from build123d import *

# Parameters (mm, degrees)
MODEL_R                 = 1.7
MODEL_R_2               = 1.600279216
MODEL_W                 = 3.1
MODEL_H                 = 6
SALIENTE_EXTRUIR1_DEPTH = 3


with BuildPart() as part:
    # Model → Saliente-Extruir1 (new body)
    with BuildSketch(Plane.XY):
        with BuildLine():
            Line((139.768153306, -45.054934941), (61.763543448, -45.054934941))
            ThreePointArc((61.763543448, -45.054934941), (60.702883276, -45.494274769), (60.263543448, -46.554934941))
            Line((60.263543448, -46.554934941), (60.263543448, -115.557339175))
            ThreePointArc((60.263543448, -115.557339175), (60.702883276, -116.617999347), (61.763543448, -117.057339175))
            Line((61.763543448, -117.057339175), (139.768153306, -117.057339175))
            ThreePointArc((139.768153306, -117.057339175), (140.828813478, -116.617999347), (141.268153306, -115.557339175))
            Line((141.268153306, -115.557339175), (141.268153306, -46.554934941))
            ThreePointArc((141.268153306, -46.554934941), (140.828813478, -45.494274769), (139.768153306, -45.054934941))
        make_face()
        with Locations((136.768487808, -103.558008179)):
            Circle(MODEL_R, mode=Mode.SUBTRACT)
        with Locations((136.768487808, -58.554600438)):
            Circle(MODEL_R, mode=Mode.SUBTRACT)
        with Locations((136.768487808, -112.557673677)):
            Circle(MODEL_R_2, mode=Mode.SUBTRACT)
        with Locations((136.768487808, -49.554934941)):
            Circle(MODEL_R_2, mode=Mode.SUBTRACT)
        with Locations((64.763543448, -103.558008179)):
            Circle(MODEL_R, mode=Mode.SUBTRACT)
        with Locations((64.763543448, -58.554600438)):
            Circle(MODEL_R, mode=Mode.SUBTRACT)
        with Locations((64.763543448, -49.554934941)):
            Circle(MODEL_R_2, mode=Mode.SUBTRACT)
        with Locations((64.763543448, -112.557673677)):
            Circle(MODEL_R_2, mode=Mode.SUBTRACT)
        with Locations((80.876831082, -110.067386969)):
            Rectangle(MODEL_W, MODEL_H, mode=Mode.SUBTRACT)
        with Locations((88.022204789, -110.067386969)):
            Rectangle(MODEL_W, MODEL_H, mode=Mode.SUBTRACT)
        Polygon((63.351345037, -62.275422733), (63.351345037, -72.689428622), (63.251345037, -72.789428622), (62.088360478, -72.789428622), (61.988360478, -72.889428622), (61.988360478, -76.624152209), (62.088360478, -76.724152209), (62.251345037, -76.724152209), (62.351345037, -76.824152209), (62.351345037, -99.677826967), (63.351345037, -99.677826967), (64.151345037, -100.477826967), (66.651345037, -100.477826967), (67.151345037, -100.977826967), (67.151345037, -114.477826967), (67.651345037, -114.977826967), (77.980472194, -114.977826967), (77.980472194, -106.277895967), (78.980472194, -105.277865819), (90.361604846, -105.277522697), (91.361604845, -106.277492548), (91.361604845, -114.977826967), (133.468205597, -114.977826967), (133.968205597, -114.477826967), (133.968205597, -100.862451961), (134.355954895, -100.477826967), (137.555954895, -100.477826967), (139.366374234, -98.667407629), (139.366374234, -61.475422733), (138.866374234, -60.975422733), (133.634687553, -60.975422733), (132.355954895, -60.088974267), (132.355954895, -48.775422733), (130.555954895, -46.975422733), (71.151345037, -46.975422733), (69.351345037, -48.775422733), (69.351345037, -58.538415371), (67.351345037, -61.475422733), (64.151345037, -61.475422733), align=None, mode=Mode.SUBTRACT)
    extrude(amount=SALIENTE_EXTRUIR1_DEPTH)


solid = part.part
Work out the finished part from the listing and answer in its coordinate system (mm). A direction names the side the tool comes from. Round coordinates to 2 decimals unless told otherwise and drop trailing zeros. Write each loop counter-clockwise with the first axis right and the second up, starting at its lowest first coordinate (ties: lowest second). Pieces come first, ordered by that corner, then holes. Notation, with made-up numbers: M 12.5,58 L 36.5,58 A21 ccw 36.5,70 Z; hole C 23,-4.5 d5. An arc over 180 degrees is marked long. Use a Markdown table: item, result.
1) The part is cut by section D-D on z = 2.1. State how many separate pieces and enclosed holes the cut face has, plus the area to 3 significant figures.
Taken from the geometry:
| item | result |
|---|---|
| separate pieces | 1 |
| enclosed holes | 11 |
| area | 977 mm2 |
2) Consider line 1 (Y direction, x = 88.5, z = 1.1); line 2 (X direction, y = -93, z = 2.6); line 3 (Y direction, x = 113, z = 0.45). Determine where each line is inside the solid, lowest interval first. Write a range as [from, to].
Taken from the geometry:
| item | result |
|---|---|
| line 1 | y = [-117.06, -113.07], [-107.07, -105.28], [-46.98, -45.05] |
| line 2 | x = [60.26, 62.35], [139.37, 141.27] |
| line 3 | y = [-117.06, -114.98], [-46.98, -45.05] |
3) Which of the six approach directions +Z, -Z, +X, -X, +Y, -Y give full straight-line access (tool end or side, diameter ignored) to faces 4 (the face through (101, -45.055, 1)), 5 (the face through (91.362, -111, 1))?
Taken from the geometry:
| item | result |
|---|---|
| face 4 | +Z, -Z, +X, -X, +Y |
| face 5 | +Z, -Z |
4) The part is cut by section B-B on y = -109. Give the vertices of the cut face in (x, z), plus the area to 3 significant figures.
Taken from the geometry:
| item | result |
|---|---|
| outline | M 60.26,0 L 67.15,0 L 67.15,3 L 60.26,3 Z; M 77.98,0 L 79.33,0 L 79.33,3 L 77.98,3 Z; M 82.43,0 L 86.47,0 L 86.47,3 L 82.43,3 Z; M 89.57,0 L 91.36,0 L 91.36,3 L 89.57,3 Z; M 133.97,0 L 141.27,0 L 141.27,3 L 133.97,3 Z |
| area | 64.1 mm2 |
5) The part is cut by section A-A on x = 96.5. Give the vertices of the cut face in (y, z).
Taken from the geometry:
| item | result |
|---|---|
| outline | M -117.06,0 L -114.98,0 L -114.98,3 L -117.06,3 Z; M -46.98,0 L -45.05,0 L -45.05,3 L -46.98,3 Z |
6) A flat-ended cylindrical pin translates along its axis: pin 1 (1.9 mm diameter, centred on x = 136.77, y = -112.56, fed in from -Z). Find the tip coordinate at first contact, or state that the pin passes through.
Taken from the geometry:
| item | result |
|---|---|
| pin 1 | passes through |
7) Determine the mould class of faces 1 (the face through (88, -107.067, 1)), 2 (the face through (101, -46, 3)), 3 (the face through (60.264, -81, 1)) for opening direction X: pulls with the +X half, pulls with the -X half, needs draft (parallel to the pull), parting line crosses it, or undercut.
Taken from the geometry:
| item | result |
|---|---|
| face 1 | undercut |
| face 2 | needs draft |
| face 3 | pulls with the -X half |
8) The part is cut by section C-C on y = -94. Give the vertices of the cut face in (x, z).
Taken from the geometry:
| item | result |
|---|---|
| outline | M 60.26,0 L 62.35,0 L 62.35,3 L 60.26,3 Z; M 139.37,0 L 141.27,0 L 141.27,3 L 139.37,3 Z |
